from build123d import *

# Parameters (mm, degrees)
F0_W      = 31.19
F0_H      = 12.93
F1_DEPTH  = 1.4
F2_R      = 1.6
F3_DEPTH  = 1.401
F4_R      = 1.5
F5_W      = 8.7
F5_H      = 3.4
F6_DEPTH  = 1.401
F7_W      = 14.75
F7_H      = 8.5
F8_DEPTH  = 19.4
F9_W      = 10.75
F9_H      = 4.5
F10_DEPTH = 19.4
F12_DEPTH = 10.716
F14_DEPTH = 9.75


with BuildPart() as f1:
    # F0 (on Top) → F1 (new body)
    with BuildSketch(Plane.XY):
        Rectangle(F0_W, F0_H)
    extrude(amount=F1_DEPTH)

    # F2 (on face) → F3 (cut, through all)
    with BuildSketch(Plane.XY.offset(1.4)):
        with Locations((-12.56, 0)):
            Circle(F2_R)
        with Locations((12.56, 0)):
            Circle(F2_R)
    extrude(amount=-F3_DEPTH, mode=Mode.SUBTRACT)

    # F4
    f4_edges = [f1.edges().sort_by_distance(p)[0] for p in [
        (15.595, -6.465, 0.7),
        (15.595, 6.465, 0.7),
        (-15.595, -6.465, 0.7),
        (-15.595, 6.465, 0.7),
    ]]
    fillet(f4_edges, radius=F4_R)

    # F5 (on face) → F6 (cut, through all)
    with BuildSketch(Plane.XY.offset(1.4)):
        Rectangle(F5_W, F5_H)
    extrude(amount=-F6_DEPTH, mode=Mode.SUBTRACT)

    # F7 (on face) → F8 (join)
    with BuildSketch(Plane.XY.offset(1.4)):
        Rectangle(F7_W, F7_H)
    extrude(amount=F8_DEPTH)

    # F9 (on face) → F10 (cut, through all)
    with BuildSketch(Plane.XY.offset(20.8)):
        Rectangle(F9_W, F9_H)
    extrude(amount=-F10_DEPTH, mode=Mode.SUBTRACT)

    # F11 (on face) → F12 (cut, through all)
    with BuildSketch(Plane.XZ.offset(4.25)):
        with BuildLine():
            Line((-4.875, 20.8), (-5.375, 20.8))
            Line((-5.375, 20.8), (-5.375, 15.05))
            ThreePointArc((-5.375, 15.05), (-5.125, 14.8), (-4.875, 15.05))
            Line((-4.875, 15.05), (-4.875, 20.8))
        make_face()
        with BuildLine():
            Line((5.375, 15.05), (5.375, 20.8))
            Line((5.375, 20.8), (4.875, 20.8))
            Line((4.875, 20.8), (4.875, 15.05))
            ThreePointArc((4.875, 15.05), (5.125, 14.8), (5.375, 15.05))
        make_face()
    extrude(amount=-F12_DEPTH, mode=Mode.SUBTRACT)

    # F13 (on face) → F14 (join, through all)
    with BuildSketch(Plane.YZ.offset(4.875)):
        Polygon((-1.55, 20.2), (-2.25, 20.8), (-2.25, 19.6), (-1.55, 19.6), align=None)
        Polygon((2.25, 19.6), (2.25, 20.8), (1.55, 20.2), (1.55, 19.6), align=None)
    extrude(amount=-F14_DEPTH)


solid = f1.part
Could you check a few things on this model? Use its own coordinates, in mm. A direction names the side the tool comes from. Coordinates: 2 decimals unless noted, no trailing zeros. Order: outer loops, then holes, each group sorted by start corner. A loop starts at its lowest first (then second) coordinate and runs counter-clockwise, first axis right, second up.
Q1. Please list where these lines run through material, in increasing order: L1, parallel to Y at x = -3.5, z = 14.5; L2, parallel to Y at x = 12.56, z = 0.3 (3 decimals); L3, parallel to X at y = -1.5, z = 19.5 (3 decimals).
Q2. Suppose I cut it at C-C on x = 3.5. Please give me the cut outline in (y, z) (3 decimals), and give its area (3 significant figures).
Q3. Thinking about a two-plate mould opening in Y: for faces 1 (the flat face through (0, 6.465, 1)), 2 (the flat face through (-4.35, 0, 1)), 3 (the flat face through (-0.2, 4.4, 1.4)), which applies, released by +Y, released by -Y, zero draft, split by the parting line, or undercut?
Q4. Suppose I cut it at D-D on z = 3.25. Please give me the cut outline in (x, y) (3 decimals).
Q5. Suppose I cut it at B-B on y = 0. Please give me the cut outline in (x, z) (3 decimals).
Q6. Will these pins go through, and if not, where does the flat tip stop? pin 1 (5 mm diameter, centred on x = 12.56, y = 0, fed in from +Z); pin 2 (12 mm diameter, centred on x = 9.5, z = 11, fed in from -Y); pin 3 (2 mm diameter, centred on x = 0, y = 1, fed in from +Z).
Q7. Suppose I cut it at A-A on z = 18. Please give me the cut outline in (x, y) (3 decimals).
Q8. Which directions (+Z, -Z, +X, -X, +Y, -Y) give clear straight access to the entire face, cutting with the end or side of a thin tool? Please do faces 4 (the flat face through (-7.375, 0, 11)), 5 (the flat face through (-5.375, 0, 13)), 6 (the flat face through (0, 1.7, 1)).
Answer:
1. L1: y = -4.25 to -2.25, 2.25 to 4.25
1. L2: y = -6.465 to -1.6, 1.6 to 6.465
1. L3: x = -7.375 to -5.375, 5.375 to 7.375
2. outline: (-6.465, 0) - (-1.7, 0) - (-1.7, 1.4) - (-2.25, 1.4) - (-2.25, 19.6) - (-1.55, 19.6) - (-1.55, 20.2) - (-2.25, 20.8) - (-4.25, 20.8) - (-4.25, 1.4) - (-6.465, 1.4) - close; (1.55, 19.6) - (2.25, 19.6) - (2.25, 1.4) - (1.7, 1.4) - (1.7, 0) - (6.465, 0) - (6.465, 1.4) - (4.25, 1.4) - (4.25, 20.8) - (2.25, 20.8) - (1.55, 20.2) - close
2. area: 92.2 mm2
3. face 1: released by +Y
3. face 2: undercut
3. face 3: zero draft
4. outline: (-7.375, -4.25) - (7.375, -4.25) - (7.375, 4.25) - (-7.375, 4.25) - close; hole (-5.375, -2.25) - (5.375, -2.25) - (5.375, 2.25) - (-5.375, 2.25) - close
5. outline: (-15.595, 0) - (-14.16, 0) - (-14.16, 1.4) - (-15.595, 1.4) - close; (-10.96, 0) - (-4.35, 0) - (-4.35, 1.4) - (-5.375, 1.4) - (-5.375, 20.8) - (-7.375, 20.8) - (-7.375, 1.4) - (-10.96, 1.4) - close; (4.35, 0) - (10.96, 0) - (10.96, 1.4) - (7.375, 1.4) - (7.375, 20.8) - (5.375, 20.8) - (5.375, 1.4) - (4.35, 1.4) - close; (14.16, 0) - (15.595, 0) - (15.595, 1.4) - (14.16, 1.4) - close
6. pin 1: stops at z = 1.4
6. pin 2: stops at y = -4.25
6. pin 3: stops at z = 20.59
7. outline: (-7.375, -4.25) - (-5.375, -4.25) - (-5.375, 4.25) - (-7.375, 4.25) - close; (-4.875, -4.25) - (4.875, -4.25) - (4.875, -2.25) - (-4.875, -2.25) - close; (-4.875, 2.25) - (4.875, 2.25) - (4.875, 4.25) - (-4.875, 4.25) - close; (5.375, -4.25) - (7.375, -4.25) - (7.375, 4.25) - (5.375, 4.25) - close
8. face 4: +Z, -X, +Y, -Y
8. face 5: +Z
8. face 6: -Z
